The listing builds one solid part. Answer for the finished solid, in the listing's coordinates (mm). Face numbers are marked on the shaded views. A direction names the side the tool comes from. Give positions to 0.01 mm unless a question says otherwise; leave off trailing zeros. Write each loop counter-clockwise with the first axis right and the second up, starting at its lowest first coordinate (ties: lowest second). Pieces come first, ordered by that corner, then holes. Notation, with made-up numbers: M 42.25,42 L 57.25,42 A8 cw 57.25,55 Z; hole C 61,72.25 d9. An arc over 180 degrees is marked long. Answer as a JSON object with one key per item and string values.
```python
from build123d import *

# Parameters (mm, degrees)
F0_W     = 1.2968151346
F0_H     = 20
F0_W_2   = 0.7031848654
F0_R     = 0.95
F2_DEPTH = 1


with BuildPart() as f1:
    # F0 (on Front) → F1 (revolve)
    with BuildSketch(Plane.XZ):
        with Locations((-12.7275561206, 21.3498084247)):
            Rectangle(F0_W, F0_H)
        with Locations((-11.7275561206, 21.3498084247)):
            Rectangle(F0_W_2, F0_H)
    revolve(axis=Axis((-15.1759636879, 0, 21.4413572103), (0, 0, -1)))

    # F0 (on Front) → F2 (join, symmetric)
    with BuildSketch(Plane.XZ):
        with Locations((-11.7275561206, 21.3498084247)):
            Rectangle(F0_W_2, F0_H)
        with BuildLine():
            Line((-5.6838793599, 31.3498084247), (-11.3759636879, 31.3498084247))
            Line((-11.3759636879, 31.3498084247), (-11.3759636879, 11.3498084247))
            Line((-11.3759636879, 11.3498084247), (-3.9564480013, 11.3498084247))
            ThreePointArc((-3.9564480013, 11.3498084247), (-2.7164166971, 11.7806295424), (-2.0106170654, 12.8874860601))
            Line((-2.0106170654, 12.8874860601), (-0.386721159, 19.7221692442))
            ThreePointArc((-0.386721159, 19.7221692442), (-0.2713600171, 21.3254265154), (-0.6706739378, 22.8824398305))
            Line((-0.6706739378, 22.8824398305), (-3.8516295355, 30.1515942946))
            ThreePointArc((-3.8516295355, 30.1515942946), (-4.5892496827, 31.0236620234), (-5.6838793599, 31.3498084247))
        make_face()
        with Locations((-3.95, 21.3498084247)):
            Circle(F0_R, mode=Mode.SUBTRACT)
    extrude(amount=F2_DEPTH, both=True)


solid = f1.part
```
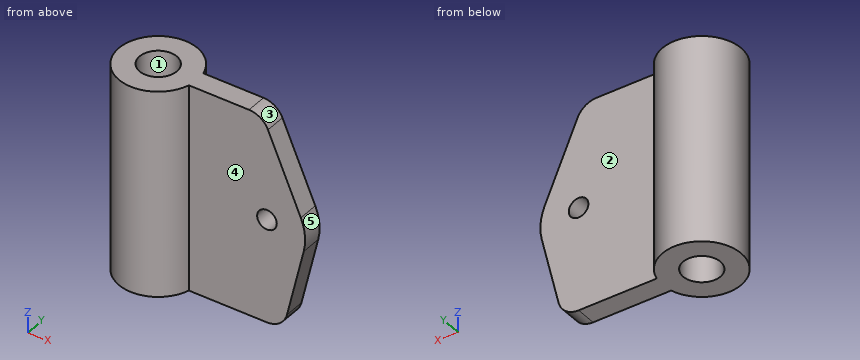
1. Flat-ended cylindrical pins translate along their axes: pin 1 (2.5 mm diameter, centred on x = -3.95, z = 21.35, fed in from -Y); pin 2 (3 mm diameter, centred on y = 2.5, z = 15.5, fed in from -X); pin 3 (9 mm diameter, centred on x = -8.5, z = 24.5, fed in from -Y). Find the tip coordinate at first contact, or state that the pin passes through.
Verdict:
{"pin 1": "stops at y = -1", "pin 2": "stops at x = -18.84", "pin 3": "stops at y = -3.12"}
2. A cutting plane is placed at B-B, the plane x = -14. Give the vertices of the cut face in (y, z), plus the area to 3 significant figures.
Verdict:
{"outline": "M -3.61,11.35 L -1.36,11.35 L -1.36,31.35 L -3.61,31.35 Z; M 1.36,11.35 L 3.61,11.35 L 3.61,31.35 L 1.36,31.35 Z", "area": "90.0 mm2"}
3. The mould has two halves that part along X. Classify the marked faces 1, 2 and 3: released by +X, released by -X, zero draft, split by the parting line, or undercut.
Verdict:
{"face 1": "undercut", "face 2": "zero draft", "face 3": "released by +X"}
4. A cutting plane is placed at A-A, the plane y = 0. Give the vertices of the cut face in (x, z).
Verdict:
{"outline": "M -18.98,11.35 L -16.98,11.35 L -16.98,31.35 L -18.98,31.35 Z; M -13.38,11.35 L -3.96,11.35 A2 ccw -2.01,12.89 L -0.39,19.72 A5 ccw -0.67,22.88 L -3.85,30.15 A2 ccw -5.68,31.35 L -13.38,31.35 Z; hole C -3.95,21.35 d1.9"}
5. A cutting plane is placed at C-C, the plane z = 17. Give the vertices of the cut face in (x, y).
Verdict:
{"outline": "M -11.51,-1 L -1.03,-1 L -1.03,1 L -11.51,1 A3.8 ccw long Z; hole C -15.18,0 d3.6"}
6. For the marked faces 4 and 5, determine the directions among +Z, -Z, +X, -X, +Y, -Y from which every point of the face is accessible in a straight line to the end or side of a thin tool.
Verdict:
{"face 4": "+Z, -Z, +X, -Y", "face 5": "+X, +Y, -Y"}
7. A cutting plane is placed at D-D, the plane y = -3. Give the vertices of the cut face in (x, z), plus the area to 3 significant figures.
Verdict:
{"outline": "M -17.51,11.35 L -12.84,11.35 L -12.84,31.35 L -17.51,31.35 Z", "area": "93.3 mm2"}
8. Consider line 1 along Y through (x, z) = (-10.75, 18); line 2 along Z through (x, y) = (-3.95, 0.5); line 3 along Y through (x, z) = (-15, 23). Determine where each line is inside the solid, lowest interval first.
Verdict:
{"line 1": "y = -1 to 1", "line 2": "z = 11.35 to 20.4, 22.3 to 30.35", "line 3": "y = -3.8 to -1.79, 1.79 to 3.8"}
